```python
from build123d import *

# Parameters (mm, degrees)
F0_W     = 250
F0_H     = 570
F1_DEPTH = 10
F3_DEPTH = 2


with BuildPart() as f1:
    # F0 (on Top) → F1 (new body)
    with BuildSketch(Plane.XY):
        with Locations((113.159475, 248.007115)):
            Rectangle(F0_W, F0_H)
    extrude(amount=F1_DEPTH)

    # F2 (on face) → F3 (join)
    with BuildSketch(Plane.XY.offset(10)):
        with BuildLine():
            ThreePointArc((174.157473, 460.044833), (43.621757, 451.505113), (52.161477, 320.969397))
            Line((52.161477, 320.969397), (55.458666, 324.728192))
            ThreePointArc((55.458666, 324.728192), (47.380553, 448.207924), (170.860284, 456.286037))
            Line((170.860284, 456.286037), (174.157473, 460.044833))
        make_face()
        with BuildLine():
            Line((55.458666, 324.728192), (52.161477, 320.969397))
            ThreePointArc((52.161477, 320.969397), (151.32972, 306.249875), (205.659475, 390.507115))
            ThreePointArc((205.659475, 390.507115), (197.416714, 428.67736), (174.157473, 460.044833))
            Line((174.157473, 460.044833), (170.860284, 456.286037))
            ThreePointArc((170.860284, 456.286037), (192.862269, 426.614103), (200.659475, 390.507115))
            ThreePointArc((200.659475, 390.507115), (149.266463, 310.804321), (55.458666, 324.728192))
        make_face()
        with BuildLine():
            ThreePointArc((205.659475, 105.507115), (197.416714, 143.67736), (174.157473, 175.044833))
            Line((174.157473, 175.044833), (170.860284, 171.286037))
            ThreePointArc((170.860284, 171.286037), (192.862269, 141.614103), (200.659475, 105.507115))
            ThreePointArc((200.659475, 105.507115), (149.266463, 25.804321), (55.458666, 39.728192))
            Line((55.458666, 39.728192), (52.161477, 35.969397))
            ThreePointArc((52.161477, 35.969397), (151.32972, 21.249875), (205.659475, 105.507115))
        make_face()
        with BuildLine():
            Line((170.860284, 171.286037), (174.157473, 175.044833))
            ThreePointArc((174.157473, 175.044833), (43.621757, 166.505113), (52.161477, 35.969397))
            Line((52.161477, 35.969397), (55.458666, 39.728192))
            ThreePointArc((55.458666, 39.728192), (47.380553, 163.207924), (170.860284, 171.286037))
        make_face()
    extrude(amount=F3_DEPTH)


solid = f1.part
```
Design review of the part built by this model. Coordinates are the model's own, in mm. A direction names the side the tool comes from. Round coordinates to 2 decimals unless told otherwise and drop trailing zeros. Order: outer loops, then holes, each group sorted by start corner. A loop starts at its lowest first (then second) coordinate and runs counter-clockwise, first axis right, second up. Notation, with made-up numbers: (37.25, -4.5) - (44.25, -4.5) arc R17 ccw to (44.25, 27.5) - close; hole circle Ø5 at (53.25, 88). An arc over 180 degrees is marked (long way). One line per question, with ' | ' between items.
Item 1: Machinability: for faces 5 (the face through (112, 107, 10)), 6 (the face through (181.2, 445.8, 12)), which of the approach directions +Z, -Z, +X, -X, +Y, -Y give a long, thin tool a straight path to every point of the face, cutting with its end or side? Answer none if there is none.
Checks:
face 5: +Z | face 6: +Z, +X, -X, +Y, -Y
Item 2: Take a section at B-B, the plane x = 92.5. Write out the cut boundary in (y, z), then the cut area to 3 significant figures.
Checks:
outline: (-36.99, 0) - (533.01, 0) - (533.01, 10) - (480.67, 10) - (480.67, 12) - (475.53, 12) - (475.53, 10) - (305.48, 10) - (305.48, 12) - (300.34, 12) - (300.34, 10) - (195.67, 10) - (195.67, 12) - (190.53, 12) - (190.53, 10) - (20.48, 10) - (20.48, 12) - (15.34, 12) - (15.34, 10) - (-36.99, 10) - close | area: 5,740 mm²
Item 3: Draft analysis for pull direction Y (two halves, no side actions). For faces 1 (the face through (111, -36.993, 5)), 2 (the face through (111, 252, 10)), 3 (the face through (111, 533.007, 5)), 4 (the face through (181.2, 160.8, 12)), state which applies: +Y half, -Y half, draft (parallel to the pull), parting line (faces both ways), or undercut.
Checks:
face 1: -Y half | face 2: undercut | face 3: +Y half | face 4: draft
Item 4: Take a section at C-C, the plane x = 213. Write out the cut boundary in (y, z).
Checks:
outline: (-36.99, 0) - (533.01, 0) - (533.01, 10) - (-36.99, 10) - close
Item 5: Take a section at D-D, the plane y = 354. Write out the cut boundary in (x, z).
Checks:
outline: (-11.84, 0) - (238.16, 0) - (238.16, 10) - (198.15, 10) - (198.15, 12) - (192.68, 12) - (192.68, 10) - (33.64, 10) - (33.64, 12) - (28.17, 12) - (28.17, 10) - (-11.84, 10) - close
Item 6: Wall thickness on line 1 (Y direction, x = 64.5, z = 11) (3 decimals); line 2 (Z direction, x = 104, y = 96): over which ranges is each line inside the solid? List them lowest first. Write a range as [from, to].
Checks:
line 1: [26.84, 32.785], [178.229, 184.174], [311.84, 317.785], [463.229, 469.174] | line 2: [0, 10]
Item 7: For P1, Ø6, axis at x = 29.5, y = 358, coming from the -Z side; P2, Ø4, axis at x = 80, y = 318.5, coming from the +Z side, all flat-tipped, find the tip position at first contact; note any pin that passes through.
Checks:
P1: z = 0 | P2: z = 10
Item 8: Take a section at A-A, the plane y = 79.5. Write out the cut boundary in (x, z), then the cut area to 3 significant figures.
Checks:
outline: (-11.84, 0) - (238.16, 0) - (238.16, 10) - (201.93, 10) - (201.93, 12) - (196.71, 12) - (196.71, 10) - (29.61, 10) - (29.61, 12) - (24.39, 12) - (24.39, 10) - (-11.84, 10) - close | area: 2,520 mm²
